```python
from build123d import *

# Parameters (mm, degrees)
PAD004_DEPTH    = 5.3
THICKNESS_T     = -2
CHAMFER_SIZE    = 1.5
SKETCH016_R     = 3
SKETCH016_R_2   = 1.65
PAD005_DEPTH    = 3.3
SKETCH018_R     = 9.5
POCKET_DEPTH    = 14
SKETCH019_R     = 14.157042
POCKET004_DEPTH = 2
SKETCH020_W     = 5
SKETCH020_H     = 1.3
POCKET005_DEPTH = 2


with BuildPart() as part:
    # Sketch015 → Pad004 (new body)
    with BuildSketch(Plane.XY):
        with BuildLine():
            Line((-2.4, 31.75), (-2.4, 0))
            ThreePointArc((-2.4, 0), (-1.697056, -1.697056), (0, -2.4))
            Line((0, -2.4), (25.4, -2.4))
            ThreePointArc((25.4, -2.4), (27.097056, -1.697056), (27.8, 0))
            Line((27.8, 0), (27.8, 31.75))
            ThreePointArc((27.8, 31.75), (27.097056, 33.447056), (25.4, 34.15))
            Line((25.4, 34.15), (0, 34.15))
            ThreePointArc((0, 34.15), (-1.697056, 33.447056), (-2.4, 31.75))
        make_face()
    extrude(amount=PAD004_DEPTH)

    # Thickness
    thickness_openings = [part.faces().sort_by_distance(p)[0] for p in [
        (12.7, 15.875, 0),
    ]]
    offset(amount=THICKNESS_T, openings=thickness_openings)

    # Chamfer
    chamfer_edges = [part.edges().sort_by_distance(p)[0] for p in [
        (-2.4, 15.875, 5.3),
    ]]
    chamfer(chamfer_edges, length=CHAMFER_SIZE)

    # Sketch016 (on Face10 of Thickness) → Pad005 (join)
    with BuildSketch(Plane(origin=(0, 0, 0), x_dir=(1, 0, 0), z_dir=(0, 0, -1))):
        with Locations((2.54, -2.54)):
            Circle(SKETCH016_R)
        with Locations((2.54, -2.54)):
            Circle(SKETCH016_R_2, mode=Mode.SUBTRACT)
        with Locations((22.86, -2.54)):
            Circle(SKETCH016_R)
        with Locations((22.86, -2.54)):
            Circle(SKETCH016_R_2, mode=Mode.SUBTRACT)
        with Locations((22.86, -29.21)):
            Circle(SKETCH016_R)
        with Locations((22.86, -29.21)):
            Circle(SKETCH016_R_2, mode=Mode.SUBTRACT)
        with Locations((2.54, -29.21)):
            Circle(SKETCH016_R)
        with Locations((2.54, -29.21)):
            Circle(SKETCH016_R_2, mode=Mode.SUBTRACT)
    extrude(amount=-PAD005_DEPTH)

    # Sketch017 (on DatumPlane) → Revolution (revolve)
    with BuildSketch(Plane.YZ.offset(12.7)):
        with BuildLine():
            Line((28.111763, 3.8), (29.111763, 3.8))
            add(Edge.make_bspline(
                [(29.111763, 3.8), (30.048452, 13.753506), (23.390882, 17.18771)],
                knots=[0, 0, 0, 1, 1, 1], degree=2))
            Line((23.390882, 17.18771), (13.782356, 17.18771))
            Line((13.782356, 17.18771), (13.782356, 16.207748))
            Line((13.782356, 16.207748), (23.191694, 16.207748))
            add(Edge.make_bspline(
                [(28.111763, 3.8), (28.400201, 12.620692), (23.191694, 16.207748)],
                knots=[0, 0, 0, 1, 1, 1], degree=2))
        make_face()
    revolve(axis=Axis((12.7, 13.782356, 17.18771), (0, 0, -1)))

    # Sketch018 (on Face6 of Revolution) → Pocket (cut)
    with BuildSketch(Plane.XY.offset(17.18771)):
        with Locations((12.7, 13.782356)):
            Circle(SKETCH018_R)
    extrude(amount=-POCKET_DEPTH, mode=Mode.SUBTRACT)

    # Sketch019 (on Face5 of Pocket) → Pocket004 (cut)
    with BuildSketch(Plane.XY.offset(5.3)):
        with Locations((12.7, 13.782356)):
            Circle(SKETCH019_R)
    extrude(amount=-POCKET004_DEPTH, mode=Mode.SUBTRACT)

    # Sketch020 (on Face25 of Pocket004) → Pocket005 (cut)
    with BuildSketch(Plane(origin=(0, 34.15, 0), x_dir=(-1, 0, 0), z_dir=(0, 1, 0))):
        with Locations((-12.662868, 0.65)):
            Rectangle(SKETCH020_W, SKETCH020_H)
    extrude(amount=-POCKET005_DEPTH, mode=Mode.SUBTRACT)


solid = part.part
```
Design review of the part built by this model. Coordinates are the model's own, in mm. A direction names the side the tool comes from. Coordinates: 2 decimals unless noted, no trailing zeros.
Q1. To check wall thickness, follow line 1 (X direction, y = 2.54, z = 1.05); line 2 (Y direction, x = 2.54, z = 1.45); line 3 (Y direction, x = 15.5, z = 1.75). State the ranges of each line that lie inside material, in increasing order.
Reported:
line 1: x = -2.4 to 0.89, 4.19 to 5.54, 19.86 to 21.21, 24.51 to 27.8
line 2: y = -2.4 to 0.89, 4.19 to 5.54, 26.21 to 27.56, 30.86 to 34.15
line 3: y = -2.4 to -0.4, 32.15 to 34.15
Q2. The part is to be moulded in two halves that separate along Y. For faces 4 (the face through (26.57, 32.9, 4.56)), 5 (the face through (26, 14, 3.3)), 6 (the face through (27, 4.3, 4.6)), say which applies: +Y half, -Y half, draft (parallel to the pull), parting line (faces both ways), or undercut.
Reported:
face 4: +Y half
face 5: undercut
face 6: draft
Q3. For pin 1 (1.6 mm diameter, centred on x = 23, y = 2, fed in from -Z); pin 2 (3.5 mm diameter, centred on x = 24, y = 2.5, fed in from +Z); pin 3 (0.6 mm diameter, centred on y = 33.5, z = 0.5, fed in from +X), all flat-tipped, find the tip position at first contact; note any pin that passes through.
Reported:
pin 1: stops at z = 3.3
pin 2: stops at z = 12.46
pin 3: stops at x = 27.31
Q4. Tool access review of faces 1 (the face through (13, -2.4, 2)), 2 (the face through (11.7, 28.1, 3.3)), 3 (the face through (21, 4, 3.3)): name each direction out of +Z, -Z, +X, -X, +Y, -Y from which nothing blocks a thin tool from reaching the whole face with its end or side.
Reported:
face 1: +Z, -Z, +X, -X, -Y
face 2: -Z
face 3: none
